```python
from build123d import *

# Parameters (mm, degrees)
SKETCH1_W           = 100
SKETCH1_H           = 70
SKETCH1_R           = 11
BOSS_EXTRUDE1_DEPTH = 5
SKETCH2_W           = 18
SKETCH2_H           = 6.5
BOSS_EXTRUDE2_DEPTH = 9
SKETCH3_R           = 2
CUT_EXTRUDE1_DEPTH  = 3
SKETCH4_R           = 3
BOSS_EXTRUDE4_DEPTH = 10
FILLET2_R           = 3
SKETCH5_R           = 2
CUT_EXTRUDE2_DEPTH  = 5


with BuildPart() as part:
    # Sketch1 → Boss-Extrude1 (new body)
    with BuildSketch(Plane(origin=(0, 0, 0), x_dir=(1, 0, 0), z_dir=(0, 1, 0))):
        Rectangle(SKETCH1_W, SKETCH1_H)
        with Locations(Location((34.5, -17.5, 0), (0, 0, 270))):
            Circle(SKETCH1_R, mode=Mode.SUBTRACT)
    extrude(amount=BOSS_EXTRUDE1_DEPTH)

    # Sketch2 → Boss-Extrude2 (add)
    with BuildSketch(Plane(origin=(0, 5, 0), x_dir=(1, 0, 0), z_dir=(0, 1, 0))):
        with BuildLine():
            Line((25.5, -35), (25.5, -23.82455532))
            ThreePointArc((25.5, -23.82455532), (34.5, -28.5), (43.5, -23.82455532))
            Line((43.5, -23.82455532), (43.5, -35))
            Line((43.5, -35), (25.5, -35))
        make_face()
        with Locations((34.5, 18.25)):
            Rectangle(SKETCH2_W, SKETCH2_H)
    extrude(amount=BOSS_EXTRUDE2_DEPTH)

    # Sketch3 → Cut-Extrude1 (cut)
    with BuildSketch(Plane(origin=(0, 14, 0), x_dir=(1, 0, 0), z_dir=(0, 1, 0))):
        with Locations(Location((29.5, -29.9, 0), (0, 0, 270))):
            Circle(SKETCH3_R)
        with Locations(Location((39.5, -29.9, 0), (0, 0, 270))):
            Circle(SKETCH3_R)
        with Locations(Location((39.5, 18.7, 0), (0, 0, 270))):
            Circle(SKETCH3_R)
        with Locations(Location((29.5, 18.7, 0), (0, 0, 270))):
            Circle(SKETCH3_R)
    extrude(amount=-CUT_EXTRUDE1_DEPTH, mode=Mode.SUBTRACT)

    # Sketch4 → Boss-Extrude4 (add)
    # profile 1 of 3: a face of its own
    with BuildSketch(Plane(origin=(0, 0, -35), x_dir=(-1, 0, 0), z_dir=(0, 0, -1))):
        Polygon((-15, -40), (15, -40), (15, -7), (15, 0), (-15, 0), (-15, -7), align=None)
        with Locations((0, -32)):
            Circle(SKETCH4_R, mode=Mode.SUBTRACT)
        with Locations((0, -8)):
            Circle(SKETCH4_R, mode=Mode.SUBTRACT)
    # profile 2 of 3: a face of its own
    with BuildSketch(Plane(origin=(0, 0, -35), x_dir=(-1, 0, 0), z_dir=(0, 0, -1))):
        Polygon((-50, 0), (-15, -7), (-15, 0), align=None)
    # profile 3 of 3: a face of its own
    with BuildSketch(Plane(origin=(0, 0, -35), x_dir=(-1, 0, 0), z_dir=(0, 0, -1))):
        Polygon((15, 0), (15, -7), (50, 0), align=None)
    extrude(amount=-BOSS_EXTRUDE4_DEPTH)

    # Fillet2
    fillet2_edges = [part.edges().sort_by_distance(p)[0] for p in [
        (15, -7, -30),
        (-15, -7, -30),
        (0, 0, -25),
    ]]
    fillet(fillet2_edges, radius=FILLET2_R)

    # Sketch5 → Cut-Extrude2 (cut)
    with BuildSketch(Plane(origin=(0, 5, 0), x_dir=(1, 0, 0), z_dir=(0, 1, 0))):
        with Locations(Location((-13.5, -30, 0), (0, 0, 270))):
            Circle(SKETCH5_R)
        with Locations(Location((-13.5, 20, 0), (0, 0, 270))):
            Circle(SKETCH5_R)
    extrude(amount=-CUT_EXTRUDE2_DEPTH, mode=Mode.SUBTRACT)


solid = part.part
```
Read the model definition and answer for the solid it produces. Units are mm, in the model's axes. A direction names the side the tool comes from. Give positions to 0.01 mm unless a question says otherwise; leave off trailing zeros. Write each loop counter-clockwise with the first axis right and the second up, starting at its lowest first coordinate (ties: lowest second). Pieces come first, ordered by that corner, then holes. Notation, with made-up numbers: (-21, -2.75) -> (24, -2.75) arc R32 cw to (24, 25.25) -> close; hole circle Ø11 at (-39.75, 2.5). An arc over 180 degrees is marked (long way). Answer in a Markdown table with one row per item.
1) Each of these flat-tipped pins is pushed along its axis until it touches: pin 1 Ø1 at (x, z) = (1.5, -1) entering from +Y; pin 2 Ø7 at (y, z) = (9.5, 31) entering from -X; pin 3 Ø2.5 at (x, z) = (39.5, -18.7) entering from -Y; pin 4 Ø3.5 at (x, y) = (0, -32) entering from +Z. Where does it stop, or does it pass through?
Results list:
| item | result |
|---|---|
| pin 1 | y = 5 |
| pin 2 | x = 25.5 |
| pin 3 | y = 0 |
| pin 4 | through |
2) Section D-D on x = -29.5 is taken. Give the vertices of the cut face in (y, z).
Results list:
| item | result |
|---|---|
| outline | (-4.1, -35) -> (5, -35) -> (5, 35) -> (0, 35) -> (0, -22) arc R3 cw to (-3, -25) -> (-4.1, -25) -> close |
3) Determine the mould class of faces 5 (the flat face through (30, 11, 30)), 6 (the flat face through (-33.5, -3.3, -30)), 7 (the cylindrical face through (28.3, 12.5, 28.3)), 8 (the flat face through (0, -40, -30)) for opening direction X: released by +X, released by -X, zero draft, split by the parting line, or undercut.
Results list:
| item | result |
|---|---|
| face 5 | undercut |
| face 6 | released by -X |
| face 7 | undercut |
| face 8 | zero draft |
4) Section B-B on x = 0 is taken. Give the vertices of the cut face in (y, z).
Results list:
| item | result |
|---|---|
| outline | (-40, -35) -> (-35, -35) -> (-35, -25) -> (-40, -25) -> close; (-29, -35) -> (-11, -35) -> (-11, -25) -> (-29, -25) -> close; (-5, -35) -> (5, -35) -> (5, 35) -> (0, 35) -> (0, -22) arc R3 cw to (-3, -25) -> (-5, -25) -> close |
5) A tool of negligible diameter and unlimited length cuts with its end or side. For faces 1 (the cylindrical face through (37.548, 12.521, -19.134)), 2 (the flat face through (-1, 0, 6)), 3 (the flat face through (25.5, 9, 29)), 4 (the flat face through (43.5, 9, -18)), from which of +Z, -Z, +X, -X, +Y, -Y can it reach the whole face along a straight path? Write none if from no direction.
Results list:
| item | result |
|---|---|
| face 1 | +Y |
| face 2 | +Z, +X, -X, -Y |
| face 3 | +Z, -Z, -X, +Y |
| face 4 | +Z, -Z, +X, +Y |
6) Section A-A on y = 7 is taken. Give the vertices of the cut face in (x, z), plus the area to 3 significant figures.
Results list:
| item | result |
|---|---|
| outline | (25.5, -21.5) -> (43.5, -21.5) -> (43.5, -15) -> (25.5, -15) -> close; (25.5, 23.82) arc R11 cw to (43.5, 23.82) -> (43.5, 35) -> (25.5, 35) -> close |
| area | 259 mm^2 |
7) Straight lines are drawn through the part: line 1 (X direction, y = 13.05, z = 29.9); line 2 (Z direction, x = 34.5, y = 6); line 3 (Y direction, x = 0, z = -27.75). For each, find the intervals that lie inside material, in ascending order. Write a range as [from, to].
Results list:
| item | result |
|---|---|
| line 1 | [25.5, 27.5], [31.5, 37.5], [41.5, 43.5] |
| line 2 | [-21.5, -15], [28.5, 35] |
| line 3 | [-40, -35], [-29, -11], [-5, 5] |
8) Section C-C on z = 12 is taken. Give the vertices of the cut face in (x, y).
Results list:
| item | result |
|---|---|
| outline | (-50, 0) -> (24.97, 0) -> (24.97, 5) -> (-50, 5) -> close; (44.03, 0) -> (50, 0) -> (50, 5) -> (44.03, 5) -> close |
